Here's how the part is built. I have some questions about the finished solid (model axes, mm). Coordinates: 2 decimals unless noted, no trailing zeros. Write each loop counter-clockwise with the first axis right and the second up, starting at its lowest first coordinate (ties: lowest second). Pieces come first, ordered by that corner, then holes. Notation, with made-up numbers: M 18,-12 L 39,-12 A27 cw 39,20 Z; hole C 57.5,-6.5 d5. An arc over 180 degrees is marked long. Use one line per item in the form item = value. Start each with the question number.
1. I want a section at A-A, the plane x = -11. List the corners of the cut face in (y, z) for me.
2. I want a section at C-C, the plane y = -127.5. List the corners of the cut face in (x, z) for me (3 decimals), plus the area to 3 significant figures.
3. I want a section at B-B, the plane z = 1068. List the corners of the cut face in (x, y) for me (3 decimals), plus the area to 3 significant figures.
4. Please list where these lines run through material, in increasing order: line 1 along Y through (x, z) = (-6.5, 10); line 2 along Z through (x, y) = (-15.5, 0); line 3 along Z through (x, y) = (13.5, -118.5). Write a range as [from, to].
5. I'm going to push flat-ended pins straight in: pin 1 Ø4 at (x, y) = (15.5, 49.5) entering from +Z; pin 2 Ø21 at (x, z) = (-2, 369) entering from -Y; pin 3 Ø6 at (x, y) = (-39, -47.5) entering from +Z. Where does each tip first touch, or does it pass through?
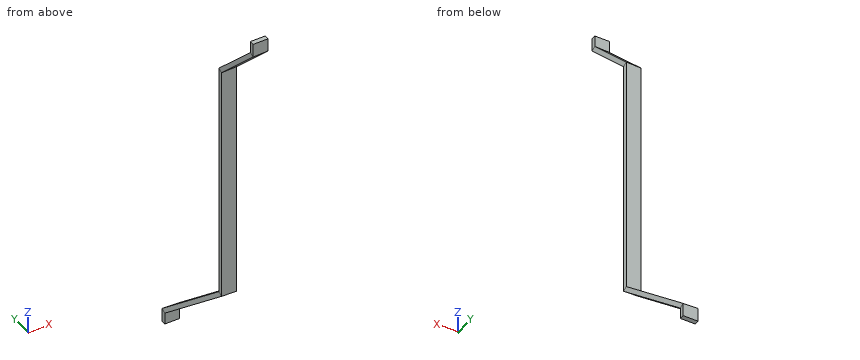
from build123d import *

# Parameters (mm, degrees)
SKETCH1_W = 70.25
SKETCH1_H = 21.6


with BuildPart() as part:
    # Sweep1: sweep along a curve in space
    with BuildLine() as sweep1_path:
        Line((-30, 400, -350), (-30, 400, -410))
        Line((0, 0, 0), (-30, 400, -350))
        Line((0, 0, 1165), (0, 0, 0))
        Line((-30, -300, 1465), (0, 0, 1165))
        Line((-30, -300, 1465), (-30, -300, 1525))
    # Sketch1 → Sweep1 (sweep)
    with BuildSketch(Plane(origin=(-30, 400, -410), x_dir=(1, 0, 0), z_dir=(0, 0, 1))):
        Rectangle(SKETCH1_W, SKETCH1_H)
    sweep(path=sweep1_path.line, transition=Transition.RIGHT)


solid = part.part
Answer list:
q1.outline = M -310.8,1461.32 L -10.8,1160.08 L -10.8,-4.52 L 389.2,-355.54 L 389.2,-410 L 410.8,-410 L 410.8,-345.75 L 10.8,5.27 L 10.8,1169.01 L -289.2,1470.25 L -289.2,1525 L -310.8,1525 Z
q2.outline = M -48.955,1306.314 L -46.795,1275.78 L 23.455,1278.686 L 21.295,1309.22 Z
q2.area = 2,150 mm²
q3.outline = M -35.125,-10.8 L 35.125,-10.8 L 35.125,10.8 L -35.125,10.8 Z
q3.area = 1,520 mm²
q4.line_1 = [-10.8, 10.8]
q4.line_2 = [-13.85, 1179.67]
q4.line_3 = [1269.24, 1299.86]
q5.pin_1 = -27.84
q5.pin_2 = -10.8
q5.pin_3 = 1229.41
